Part model, mm, in its own coordinate system. Coordinates: 2 decimals unless noted, no trailing zeros. Answer in a Markdown table with one row per item. Add a question column.
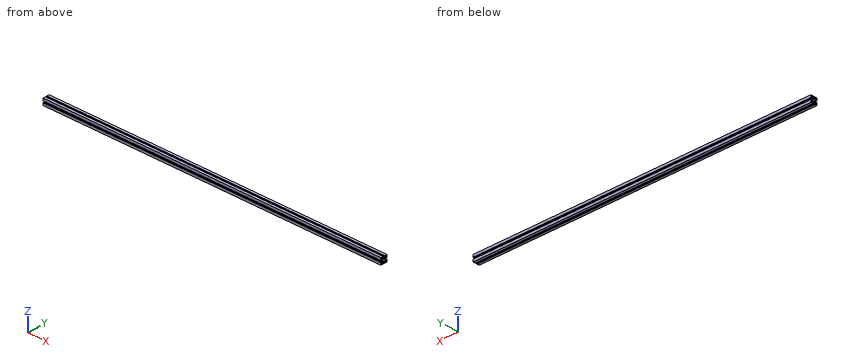
Autodesk Inventor part; units mm, degrees
ref_plane "YZ Plane" through (0, 0, 0) normal (1, 0, 0) x (0, 1, 0)
ref_plane "XZ Plane" through (0, 0, 0) normal (0, 1, 0) x (-1, 0, 0)
ref_plane "XY Plane" through (0, 0, 0) normal (0, 0, 1) x (1, 0, 0)
sketch "Skizze_1" plane through (0, 0, 0) normal (1, 0, 0) x (0, 1, 0)
  line L0 (0, 0) -> (0, -9.475)
  line L1 (0, -9.475) -> (2, -9.475)
  line L2 (2, -9.475) -> (2, -7.25)
  line L3 (2, -7.25) -> (5.5, -7.25)
  line L4 (5.5, -7.25) -> (6.5, -8.25)
  line L5 (6.5, -8.25) -> (6.5, -16.75)
  line L6 (6.5, -16.75) -> (5.5, -17.75)
  line L7 (5.5, -17.75) -> (2, -17.75)
  line L8 (2, -17.75) -> (2, -15.525)
  line L9 (2, -15.525) -> (0, -15.525)
  line L10 (0, -15.525) -> (0, -25)
  line L11 (0, -25) -> (9.475, -25)
  line L12 (9.475, -25) -> (9.475, -23)
  line L13 (9.475, -23) -> (7.25, -23)
  line L14 (7.25, -23) -> (7.25, -19.5)
  line L15 (7.25, -19.5) -> (8.25, -18.5)
  line L16 (8.25, -18.5) -> (16.75, -18.5)
  line L17 (16.75, -18.5) -> (17.75, -19.5)
  line L18 (17.75, -19.5) -> (17.75, -23)
  line L19 (17.75, -23) -> (15.525, -23)
  line L20 (15.525, -23) -> (15.525, -25)
  line L21 (15.525, -25) -> (25, -25)
  line L22 (25, -25) -> (25, -15.525)
  line L23 (25, -15.525) -> (23, -15.525)
  line L24 (23, -15.525) -> (23, -17.75)
  line L25 (23, -17.75) -> (19.5, -17.75)
  line L26 (19.5, -17.75) -> (18.5, -16.75)
  line L27 (18.5, -16.75) -> (18.5, -8.25)
  line L28 (18.5, -8.25) -> (19.5, -7.25)
  line L29 (19.5, -7.25) -> (23, -7.25)
  line L30 (23, -7.25) -> (23, -9.475)
  line L31 (23, -9.475) -> (25, -9.475)
  line L32 (25, -9.475) -> (25, 0)
  line L33 (25, 0) -> (15.525, 0)
  line L34 (15.525, 0) -> (15.525, -2)
  line L35 (15.525, -2) -> (17.75, -2)
  line L36 (17.75, -2) -> (17.75, -5.5)
  line L37 (17.75, -5.5) -> (16.75, -6.5)
  line L38 (16.75, -6.5) -> (8.25, -6.5)
  line L39 (8.25, -6.5) -> (7.25, -5.5)
  line L40 (7.25, -5.5) -> (7.25, -2)
  line L41 (7.25, -2) -> (9.475, -2)
  line L42 (9.475, -2) -> (9.475, 0)
  line L43 (9.475, 0) -> (0, 0)
  circle A0 centre (3.75, -21.25) radius 2.1
  circle A1 centre (21.25, -21.25) radius 2.1
  circle A2 centre (12.5, -12.5) radius 4.25
  circle A3 centre (3.75, -3.75) radius 2.1
  circle A4 centre (21.25, -3.75) radius 2.1
extrude "Extrusion1" add sketch "Skizze_1" along normal blind 1300
equation "\"d0\" = L"
equation "\"L\" = 1300"
properties part number "25.01.1300(00-00-0)(0)"
(1) Slice it at A-A (x = 527). State how many separate pieces and enclosed holes the cut face has, and give its area (3 significant figures).
(2) Wall check: line 1 (Z direction, x = 394.5, y = 21.25); line 2 (Y direction, x = 1122, z = -20.5); line 3 (Y direction, x = 1213, z = -11.75). Give the ranges that are in metal, low to high.
(3) Drop flat-ended pins along their axis: P1, Ø6, axis at x = 194.5, z = -11.5, coming from the -Y side; P2, Ø2, axis at x = 913.5, y = 11.5, coming from the +Z side. Give the stop position or say it passes through.
Computed:
| question | item | result |
|---|---|---|
| 1 | separate pieces | 1 |
| 1 | enclosed holes | 5 |
| 1 | area | 279 mm^2 |
| 2 | line 1 | z = -25 to -23.35, -19.15 to -17.75, -7.25 to -5.85, -1.65 to 0 |
| 2 | line 2 | y = 0 to 1.79, 5.71 to 7.25, 17.75 to 19.29, 23.21 to 25 |
| 2 | line 3 | y = 6.5 to 8.32, 16.68 to 18.5 |
| 3 | P1 | stops at y = 0 |
| 3 | P2 | stops at z = -6.5 |
